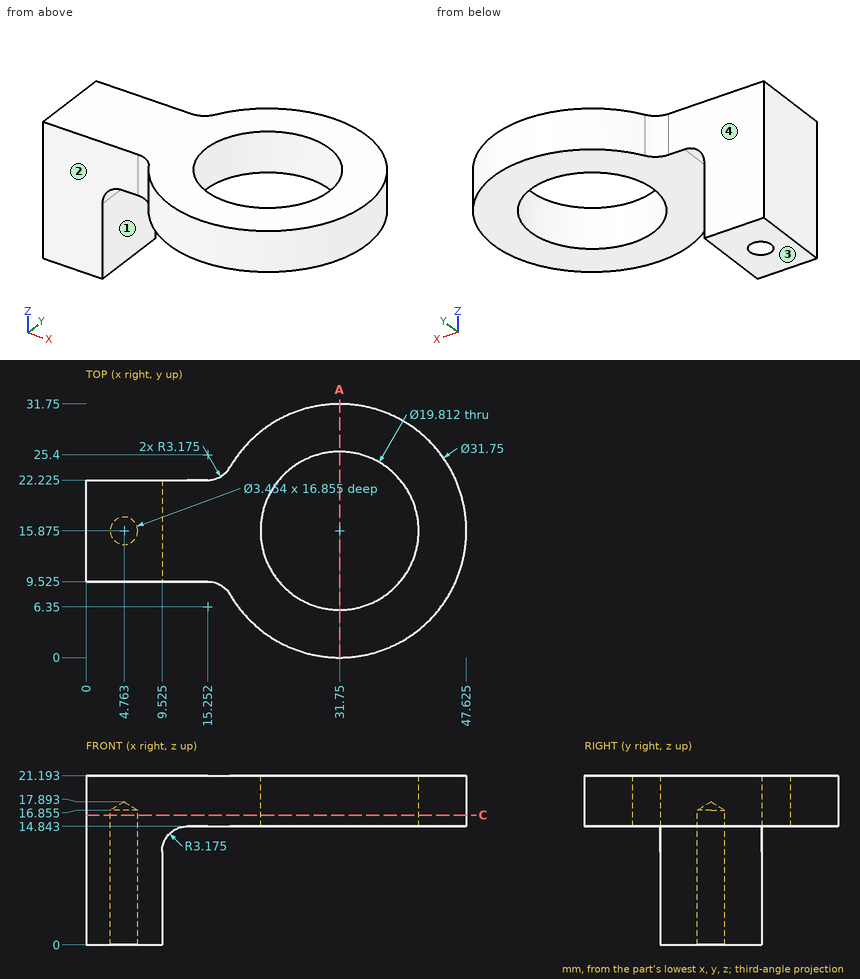
Geometry: see drawing. Coordinates: mm, zero at the bounding-box minimum. A direction names the side the tool comes from. Round coordinates to 2 decimals unless told otherwise and drop trailing zeros. Loops run counter-clockwise (first coordinate to the right, second up) from the corner with the lowest first, then second, coordinate; pieces in that order, holes last. Notation, with made-up numbers: (50, 74) -> (106, 74) arc R22 cw to (106, 91) -> close; hole circle Ø4 at (72, -10.5). An arc over 180 degrees is marked (long way). Use one line per item in the form item = value. Start each with the question number.
Item 1: Material intervals for L1, parallel to Z at x = 18, y = 16; L2, parallel to Y at x = 9.5, z = 20.25 (1 decimal); L3, parallel to Y at x = 3.5, z = 2.75 (1 decimal), sorted ascending. Write a range as from..to.
Item 2: Section query C-C on z = 16.25. Count the separate pieces of the cut face and the enclosed holes in it.
Item 3: Contact query for flat-ended pins moving along their axis: pin 1 Ø6 at (y, z) = (13, 7) entering from +X (1 decimal); pin 2 Ø2 at (x, y) = (34.5, 5) entering from -Z; pin 3 Ø7.5 at (x, z) = (4, 6) entering from +Y (1 decimal). Output: stop coordinate, or through.
Item 4: Set-up query: the marked faces 1, 2, 3 and 4. Return all of +Z, -Z, +X, -X, +Y, -Y with unobstructed straight access to the full face (end or side cutting, diameter ignored); none if empty.
Item 5: Section query A-A on x = 31.75. Return the cut outline in (y, z).
Ans:
q1.L1 = 14.84..21.19
q1.L2 = 9.5..22.2
q1.L3 = 9.5..14.7, 17.1..22.2
q2.separate_pieces = 1
q2.enclosed_holes = 2
q3.pin_1 = 9.5
q3.pin_2 = 14.84
q3.pin_3 = 22.2
q4.face_1 = -Z, +X, +Y, -Y
q4.face_2 = +Z, -Z, -X, -Y
q4.face_3 = -Z, +X, -X, +Y, -Y
q4.face_4 = +Z, -Z, -X, +Y
q5.outline = (0, 14.84) -> (5.97, 14.84) -> (5.97, 21.19) -> (0, 21.19) -> close; (25.78, 14.84) -> (31.75, 14.84) -> (31.75, 21.19) -> (25.78, 21.19) -> close
